```python
from build123d import *

# Parameters (mm, degrees)
SKETCH_1_W          = 50
SKETCH_1_H          = 225
EXTRUDE_1_DEPTH     = 25
SKETCH_2_R          = 10.5
CUT_EXTRUDE_1_DEPTH = 26
CHAMFER_1_SIZE      = 1


with BuildPart() as part:
    # Эскиз1 → Бобышка-Вытянуть1 (new body)
    with BuildSketch(Plane.XY):
        with Locations((25, 112.5)):
            Rectangle(SKETCH_1_W, SKETCH_1_H)
    extrude(amount=EXTRUDE_1_DEPTH)

    # Эскиз2 → Вырез-Вытянуть1 (cut, through all)
    with BuildSketch(Plane.XY.offset(25)):
        with Locations((25, 200)):
            Circle(SKETCH_2_R)
        with BuildLine():
            Line((14.5, 25), (14.5, 150))
            ThreePointArc((14.5, 150), (25, 160.5), (35.5, 150))
            Line((35.5, 150), (35.5, 25))
            ThreePointArc((35.5, 25), (25, 14.5), (14.5, 25))
        make_face()
    extrude(amount=-CUT_EXTRUDE_1_DEPTH, mode=Mode.SUBTRACT)

    # Фаска1
    chamfer_1_edges = [part.edges().sort_by_distance(p)[0] for p in [
        (25, 14.5, 0),
        (14.5, 87.5, 0),
        (25, 160.5, 0),
        (35.5, 87.5, 0),
        (25, 14.5, 25),
        (35.5, 87.5, 25),
        (25, 160.5, 25),
        (14.5, 87.5, 25),
        (14.5, 200, 0),
        (14.5, 200, 25),
    ]]
    chamfer(chamfer_1_edges, length=CHAMFER_1_SIZE)


solid = part.part
```
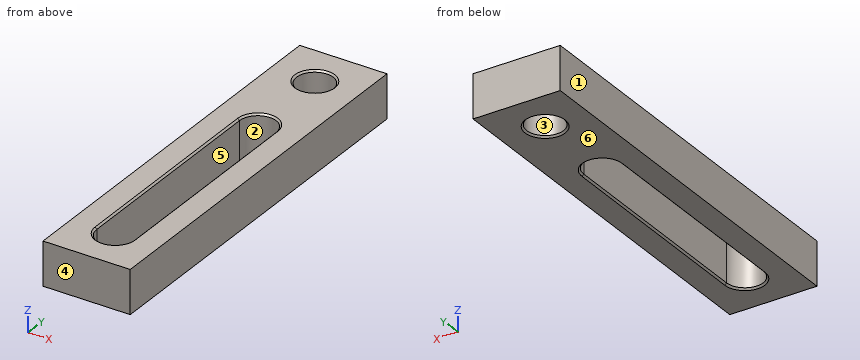
Build history of the part. All positions in model axes, mm. Face numbers are marked on the shaded views. A direction names the side the tool comes from. Give positions to 0.01 mm unless a question says otherwise; leave off trailing zeros. Order: outer loops, then holes, each group sorted by start corner. A loop starts at its lowest first (then second) coordinate and runs counter-clockwise, first axis right, second up. Notation, with made-up numbers: M 42.25,-4.75 L 81.25,-4.75 A20 cw 81.25,22.25 Z; hole C 26.5,-39.75 d9. An arc over 180 degrees is marked long. Return JSON: item names as keys, results as strings.
Q1. Band-saw the part on B-B (x = 25). Give the cut face in (y, z).
Answer list:
{"outline": "M 0,0 L 13.5,0 L 14.5,1 L 14.5,24 L 13.5,25 L 0,25 Z; M 160.5,1 L 161.5,0 L 188.5,0 L 189.5,1 L 189.5,24 L 188.5,25 L 161.5,25 L 160.5,24 Z; M 210.5,1 L 211.5,0 L 225,0 L 225,25 L 211.5,25 L 210.5,24 Z"}
Q2. Wall check: probe 1 along X at (y, z) = (149, 18); probe 2 along Y at (x, z) = (24.5, 19.5); probe 3 along Y at (x, z) = (27.5, 3.75). Give the ranges that are in metal, low to high. Write a range as from..to.
Answer list:
{"probe 1": "x = 0..14.5, 35.5..50", "probe 2": "y = 0..14.51, 160.49..189.51, 210.49..225", "probe 3": "y = 0..14.8, 160.2..189.8, 210.2..225"}
Q3. 3-axis set-ups, long thin cutter, end or side, ignore diameter. For the marked faces 1 and 2: which of +Z, -Z, +X, -X, +Y, -Y reach the whole face in a straight line?
Answer list:
{"face 1": "+Z, -Z, -X, +Y, -Y", "face 2": "+Z, -Z"}
Q4. Two-plate mould, pull along Y, no slides. Class the marked faces 3, 4, 5 and 6: pulls with the +Y half, pulls with the -Y half, needs draft (parallel to the pull), parting line crosses it, or undercut.
Answer list:
{"face 3": "undercut", "face 4": "pulls with the -Y half", "face 5": "undercut", "face 6": "needs draft"}
Q5. Band-saw the part on A-A (y = 200). Give the cut face in (x, z).
Answer list:
{"outline": "M 0,0 L 13.5,0 L 14.5,1 L 14.5,24 L 13.5,25 L 0,25 Z; M 35.5,1 L 36.5,0 L 50,0 L 50,25 L 36.5,25 L 35.5,24 Z"}
Q6. Band-saw the part on C-C (z = 9.5). Give the cut face in (x, y).
Answer list:
{"outline": "M 0,0 L 50,0 L 50,225 L 0,225 Z; hole M 14.5,25 A10.5 ccw 35.5,25 L 35.5,150 A10.5 ccw 14.5,150 Z; hole C 25,200 d21"}
